Check sheet for the modelled part. Datum: model origin and axes. Units: mm. A direction names the side the tool comes from. Round coordinates to 2 decimals unless told otherwise and drop trailing zeros. Write each loop counter-clockwise with the first axis right and the second up, starting at its lowest first coordinate (ties: lowest second). Pieces come first, ordered by that corner, then holes.
Item 1: Material ranges on line 1 (Y direction, x = 0, z = 1.5); line 2 (Y direction, x = 0, z = 2.8); line 3 (X direction, y = -17.5, z = 3.75), recorded low to high.
Item 2: Release check for a two-part mould opening along Y. For faces 3 (the flat face through (0, -20, 2)), 4 (the cylindrical face through (0, -16, 1)), 5 (the flat face through (0, 0, 5)) record: +Y half, -Y half, draft (parallel to the pull), parting line (faces both ways), or undercut.
Item 3: Cross-section at B-B on x = 0. Enter the section's corners in (y, z).
Item 4: Cross-section at C-C on z = 4.5. Enter the section's corners in (x, y).
Item 5: Cross-section at A-A on y = 17.5. Enter the section's corners in (x, z), plus the area to 3 significant figures.
Item 6: Cross-section at D-D on z = 0.95. Enter the section's corners in (x, y), plus the area to 3 significant figures.
Item 7: Tool access check on faces 1 (the cylindrical face through (-0.26, -15.517, 3.479)), 2 (the flat face through (-3.5, 0, 2)). Record the directions out of +Z, -Z, +X, -X, +Y, -Y that give a thin tool (end or side, any length) a straight path to the whole face; none if there is none.
from build123d import *

# Parameters (mm, degrees)
SKETCH1_W           = 7
SKETCH1_H           = 40
SKETCH1_R           = 2
BOSS_EXTRUDE1_DEPTH = 5
SKETCH3_R           = 2.25
BOSS_EXTRUDE2_DEPTH = 2
SKETCH4_R           = 1.5
CUT_EXTRUDE1_DEPTH  = 2


with BuildPart() as part:
    # Sketch1 → Boss-Extrude1 (new body)
    with BuildSketch(Plane.XY):
        Rectangle(SKETCH1_W, SKETCH1_H)
        with Locations((0, 17.5)):
            Circle(SKETCH1_R, mode=Mode.SUBTRACT)
        with Locations((0, -17.5)):
            Circle(SKETCH1_R, mode=Mode.SUBTRACT)
    extrude(amount=BOSS_EXTRUDE1_DEPTH)

    # Sketch3 → Boss-Extrude2 (add)
    with BuildSketch(Plane(origin=(0, 0, 0), x_dir=(-1, 0, 0), z_dir=(0, 0, -1))):
        with Locations((0, -17.5)):
            Circle(SKETCH3_R)
    extrude(amount=-BOSS_EXTRUDE2_DEPTH)

    # Sketch4 → Cut-Extrude1 (cut)
    with BuildSketch(Plane.XY.offset(2)):
        with Locations((0, -17.5)):
            Circle(SKETCH4_R)
    extrude(amount=-CUT_EXTRUDE1_DEPTH, mode=Mode.SUBTRACT)


solid = part.part
Response values:
1. line 1: y = -20 to -19, -16 to 15.5, 19.5 to 20
1. line 2: y = -20 to -19.5, -15.5 to 15.5, 19.5 to 20
1. line 3: x = -3.5 to -2, 2 to 3.5
2. face 3: -Y half
2. face 4: undercut
2. face 5: draft
3. outline: (-20, 0) - (-19, 0) - (-19, 2) - (-19.5, 2) - (-19.5, 5) - (-20, 5) - close; (-16, 0) - (15.5, 0) - (15.5, 5) - (-15.5, 5) - (-15.5, 2) - (-16, 2) - close; (19.5, 0) - (20, 0) - (20, 5) - (19.5, 5) - close
4. outline: (-3.5, -20) - (3.5, -20) - (3.5, 20) - (-3.5, 20) - close; hole circle Ø4 at (0, -17.5); hole circle Ø4 at (0, 17.5)
5. outline: (-3.5, 0) - (-2, 0) - (-2, 5) - (-3.5, 5) - close; (2, 0) - (3.5, 0) - (3.5, 5) - (2, 5) - close
5. area: 15.0 mm2
6. outline: (-3.5, -20) - (3.5, -20) - (3.5, 20) - (-3.5, 20) - close; hole circle Ø4 at (0, 17.5); hole circle Ø3 at (0, -17.5)
6. area: 260 mm2
7. face 1: +Z
7. face 2: +Z, -Z, -X, +Y, -Y
